```python
from build123d import *

# Parameters (mm, degrees)
SKETCH_1_R      = 5
EXTRUDE_1_DEPTH = 5
SKETCH_1_3_W    = 5
SKETCH_1_3_H    = 5
EXTRUDE_2_DEPTH = 10
SKETCH_1_4_W    = 5
SKETCH_1_4_H    = 15
EXTRUDE_3_DEPTH = 15


with BuildPart() as part:
    # 草圖1 → 填料-伸長1 (new body)
    with BuildSketch(Plane(origin=(0, 0, 0), x_dir=(1, 0, 0), z_dir=(0, 1, 0))):
        with BuildLine():
            ThreePointArc((0, -10), (10, 0), (0, 10))
            Line((0, 10), (-10, 10))
            Line((-10, 10), (-10, -5))
            Line((-10, -5), (-10, -10))
            Line((-10, -10), (0, -10))
        make_face()
        Circle(SKETCH_1_R, mode=Mode.SUBTRACT)
    extrude(amount=EXTRUDE_1_DEPTH)

    # 草圖1<3> → 填料-伸長2 (add)
    with BuildSketch(Plane(origin=(0, 0, 0), x_dir=(1, 0, 0), z_dir=(0, 1, 0))):
        with Locations((-12.5, -7.5)):
            Rectangle(SKETCH_1_3_W, SKETCH_1_3_H)
    extrude(amount=EXTRUDE_2_DEPTH)

    # 草圖1<4> → 填料-伸長3 (add)
    with BuildSketch(Plane(origin=(0, 0, 0), x_dir=(1, 0, 0), z_dir=(0, 1, 0))):
        with Locations((-12.5, 2.5)):
            Rectangle(SKETCH_1_4_W, SKETCH_1_4_H)
    extrude(amount=EXTRUDE_3_DEPTH)


solid = part.part
```
Geometry: final body of the model. Coordinates: model frame, mm. A direction names the side the tool comes from. Coordinates: 2 decimals unless noted, no trailing zeros. Loops run counter-clockwise (first coordinate to the right, second up) from the corner with the lowest first, then second, coordinate; pieces in that order, holes last. Notation, with made-up numbers: M 46,47.5 L 96,47.5 A20 cw 96,57.5 Z; hole C 32.25,-7.75 d4. An arc over 180 degrees is marked long. Put each result on its own line as item: value.
(1) Draft query along Z for faces 1 (the face through (10, 2, 0)), 2 (the face through (-13, 15, -3)), 3 (the face through (-1.08, 2.46, 4.88)). Return one class per face: pulls with the +Z half, pulls with the -Z half, needs draft (parallel to the pull), parting line crosses it, or undercut.
Answer sheet:
face 1: parting line crosses it
face 2: needs draft
face 3: undercut
(2) Access query for faces 4 (the face through (-9, 4, -10)), 5 (the face through (-5, 5, 2)), 6 (the face through (-13, 12, 5)). Directions: +Z, -Z, +X, -X, +Y, -Y. A direction counts if a zero-diameter tool reaches every point of the face in a straight line with its end or side. Return the directions, or none.
Answer sheet:
face 4: -Z, +X, -X, +Y, -Y
face 5: +Z, -Z, +X, +Y
face 6: +Z, +X, -X, +Y
(3) Material intervals for probe 1 along X at (y, z) = (4.05, 0); probe 2 along Y at (x, z) = (-8.75, 3); probe 3 along X at (y, z) = (12.75, 3), sorted ascending.
Answer sheet:
probe 1: x = -15 to -5, 5 to 10
probe 2: y = 0 to 5
probe 3: x = -15 to -10
(4) Cut plane C-C on z = 6. Return the cut outline in (x, y), then the cut area to 3 significant figures.
Answer sheet:
outline: M -15,0 L 8,0 L 8,5 L -10,5 L -10,10 L -15,10 Z
area: 140 mm^2
(5) First-contact query: pin 1 (5 mm diameter, centred on x = 3, y = 5.5, fed in from +Z); pin 2 (3 mm diameter, centred on y = 8.5, z = 1.5, fed in from +X); pin 3 (2.5 mm diameter, centred on x = -12, z = 7, fed in from +Y). Flat tips, straight axial feed; report the tip coordinate or a pass-through.
Answer sheet:
pin 1: stops at z = 9.98
pin 2: stops at x = -10
pin 3: stops at y = 10
(6) Cut plane D-D on x = -13. Return the cut outline in (y, z), then the cut area to 3 significant figures.
Answer sheet:
outline: M 0,-10 L 15,-10 L 15,5 L 10,5 L 10,10 L 0,10 Z
area: 275 mm^2
(7) Cut plane A-A on z = 0. Return the cut outline in (x, y), then the cut area to 3 significant figures.
Answer sheet:
outline: M -15,0 L -5,0 L -5,5 L -10,5 L -10,15 L -15,15 Z; M 5,0 L 10,0 L 10,5 L 5,5 Z
area: 125 mm^2
(8) Cut plane B-B on y = 1.5. Return the cut outline in (x, z).
Answer sheet:
outline: M -15,-10 L 0,-10 A10 ccw 0,10 L -15,10 Z; hole C 0,0 d10
